from build123d import *

# Parameters (mm, degrees)
SKETCH1_R                 = 1.1
BOSS_EXTRUDE1_DEPTH       = 5
SKETCH2_W                 = 31
SKETCH2_H                 = 2
CUT_EXTRUDE1_DEPTH        = 22
SKETCH4_R                 = 5
BOSS_EXTRUDE2_DEPTH       = 5
F_1_5MM_DOWEL_HOLE1_D     = 1.5
F_1_5MM_DOWEL_HOLE1_DEPTH = 5


with BuildPart() as part:
    # Sketch1 → Boss-Extrude1 (new body)
    with BuildSketch(Plane.XY):
        with BuildLine():
            Line((-10.5, 9.35), (-17.5, 9.35))
            Line((-17.5, 9.35), (-17.5, -23.65))
            Line((-17.5, -23.65), (-2.5, -23.65))
            Line((-2.5, -23.65), (-2.5, -38.65))
            Line((-2.5, -38.65), (2.5, -38.65))
            Line((2.5, -38.65), (2.5, -23.65))
            Line((2.5, -23.65), (17.5, -23.65))
            Line((17.5, -23.65), (17.5, 9.35))
            Line((17.5, 9.35), (10.5, 9.35))
            ThreePointArc((10.5, 9.35), (7.4, 6.25), (10.5, 3.15))
            Line((10.5, 3.15), (13.5, 3.15))
            Line((13.5, 3.15), (13.5, -3.15))
            Line((13.5, -3.15), (10.5, -3.15))
            ThreePointArc((10.5, -3.15), (7.4, -6.25), (10.5, -9.35))
            Line((10.5, -9.35), (13.5, -9.35))
            Line((13.5, -9.35), (13.5, -18.75))
            Line((13.5, -18.75), (-13.5, -18.75))
            Line((-13.5, -18.75), (-13.5, -9.35))
            Line((-13.5, -9.35), (-10.5, -9.35))
            ThreePointArc((-10.5, -9.35), (-7.4, -6.25), (-10.5, -3.15))
            Line((-10.5, -3.15), (-13.5, -3.15))
            Line((-13.5, -3.15), (-13.5, 3.15))
            Line((-13.5, 3.15), (-10.5, 3.15))
            ThreePointArc((-10.5, 3.15), (-7.4, 6.25), (-10.5, 9.35))
        make_face()
        with Locations((-10.5, 6.25)):
            Circle(SKETCH1_R, mode=Mode.SUBTRACT)
        with Locations((10.5, 6.25)):
            Circle(SKETCH1_R, mode=Mode.SUBTRACT)
        with Locations((10.5, -6.25)):
            Circle(SKETCH1_R, mode=Mode.SUBTRACT)
        with Locations((-10.5, -6.25)):
            Circle(SKETCH1_R, mode=Mode.SUBTRACT)
    extrude(amount=BOSS_EXTRUDE1_DEPTH)

    # Sketch2 → Cut-Extrude1 (cut)
    with BuildSketch(Plane(origin=(0, 9.35, 0), x_dir=(1, 0, 0), z_dir=(0, 1, 0))):
        with Locations((0, -2.5)):
            Rectangle(SKETCH2_W, SKETCH2_H)
    extrude(amount=-CUT_EXTRUDE1_DEPTH, mode=Mode.SUBTRACT)

    # Sketch4 → Boss-Extrude2 (add)
    with BuildSketch(Plane.XZ.offset(38.65)):
        with Locations(Location((0, 2.5, 0), (0, 0, 270))):
            Circle(SKETCH4_R)
    extrude(amount=BOSS_EXTRUDE2_DEPTH)

    # Ø1.5mm Dowel Hole1
    with Locations(Plane(origin=(3.75, -38.65, 2.5), x_dir=(0, 0, 1), z_dir=(0, 1, 0))):
        with Locations((0, 0), (0, -7.5)):
            Hole(F_1_5MM_DOWEL_HOLE1_D / 2, depth=F_1_5MM_DOWEL_HOLE1_DEPTH)


solid = part.part
Part model, mm, in its own coordinate system. A direction names the side the tool comes from. Give positions to 0.01 mm unless a question says otherwise; leave off trailing zeros. Write each loop counter-clockwise with the first axis right and the second up, starting at its lowest first coordinate (ties: lowest second). Pieces come first, ordered by that corner, then holes.
1) Two-plate mould, pull along X, no slides. Class faces 4 (the face through (2.5, -31, 2)), 5 (the face through (10, -23.65, 2)), 6 (the face through (-15, -12.65, 2)), 7 (the face through (3.018, -41.185, 2.663)): released by +X, released by -X, zero draft, split by the parting line, or undercut.
Resolved:
face 4: released by +X
face 5: zero draft
face 6: undercut
face 7: undercut
2) Cut at B-B on z = 2.5. Write the cut outline in (x, y).
Resolved:
outline: (-17.5, -23.65) - (-2.5, -23.65) - (-2.5, -38.65) - (-3, -38.65) - (-3, -43.65) - (3, -43.65) - (3, -38.65) - (2.5, -38.65) - (2.5, -23.65) - (17.5, -23.65) - (17.5, 9.35) - (15.5, 9.35) - (15.5, -12.65) - (13.5, -12.65) - (13.5, -18.75) - (-13.5, -18.75) - (-13.5, -12.65) - (-15.5, -12.65) - (-15.5, 9.35) - (-17.5, 9.35) - close; (-5, -43.65) - (-4.5, -43.65) - (-4.5, -38.65) - (-5, -38.65) - close; (4.5, -43.65) - (5, -43.65) - (5, -38.65) - (4.5, -38.65) - close
3) Which spindle directions (+Z, -Z, +X, -X, +Y, -Y) get a long thin tool onto all of the face, cutting with end or side? Do faces 1 (the face through (-14, -1, 3.5)), 2 (the face through (-2.5, -31, 2)), 3 (the face through (12, -9.35, 4)). Say none if no direction does.
Resolved:
face 1: +Y
face 2: +Z, -Z, -X
face 3: +Z, -Z
4) Probe L1, parallel to Y at x = 13, z = 4.75; L2, parallel to Y at x = 10.5, z = 4.65; L3, parallel to X at y = -41.2, z = 2.5. List the from-to ranges inside material, lowest first.
Resolved:
L1: y = -23.65 to -18.75, -9.35 to -3.15, 3.15 to 9.35
L2: y = -23.65 to -18.75, -9.35 to -7.35, -5.15 to -3.15, 3.15 to 5.15, 7.35 to 9.35
L3: x = -5 to -4.5, -3 to 3, 4.5 to 5
5) Cut at A-A on y = 6.25. State how many separate pieces and enclosed holes the cut face has, then the cut area to 3 significant figures.
Resolved:
separate pieces: 6
enclosed holes: 0
area: 55.4 mm2
6) Pin check, flat tips, straight feed: pin 1 (12 mm diameter, centred on x = 10, y = -8.5, fed in from +Z); pin 2 (3 mm diameter, centred on x = 6, z = 2.5, fed in from -Y); pin 3 (5.5 mm diameter, centred on y = -31.5, z = 3, fed in from +X); pin 4 (4 mm diameter, centred on x = -10.5, y = 1.5, fed in from -Z). Stop position of each tip, or through.
Resolved:
pin 1: stops at z = 5
pin 2: stops at y = -43.65
pin 3: stops at x = 2.5
pin 4: stops at z = 0
7) Cut at D-D on x = 0. Write the cut outline in (y, z), then the cut area to 4 significant figures.
Resolved:
outline: (-43.65, -2.5) - (-38.65, -2.5) - (-38.65, 0) - (-18.75, 0) - (-18.75, 5) - (-38.65, 5) - (-38.65, 7.5) - (-43.65, 7.5) - close
area: 149.5 mm2
8) Cut at C-C on x = -3.75. Write the cut outline in (y, z), then the cut area to 3 significant figures.
Resolved:
outline: (-43.65, -0.81) - (-38.65, -0.81) - (-38.65, 1.75) - (-43.65, 1.75) - close; (-43.65, 3.25) - (-38.65, 3.25) - (-38.65, 5.81) - (-43.65, 5.81) - close; (-23.65, 0) - (-18.75, 0) - (-18.75, 5) - (-23.65, 5) - close
area: 50.1 mm2
